Design review of the part built by this model. Coordinates are the model's own, in mm. Give positions to 0.01 mm unless a question says otherwise; leave off trailing zeros. Order: outer loops, then holes, each group sorted by start corner. A loop starts at its lowest first (then second) coordinate and runs counter-clockwise, first axis right, second up. Notation, with made-up numbers: (-4, -25.75) -> (5, -25.75) arc R26 cw to (5, -11.75) -> close; hole circle Ø8 at (72.25, 59.5). An arc over 180 degrees is marked (long way). Return JSON: item names as keys, results as strings.
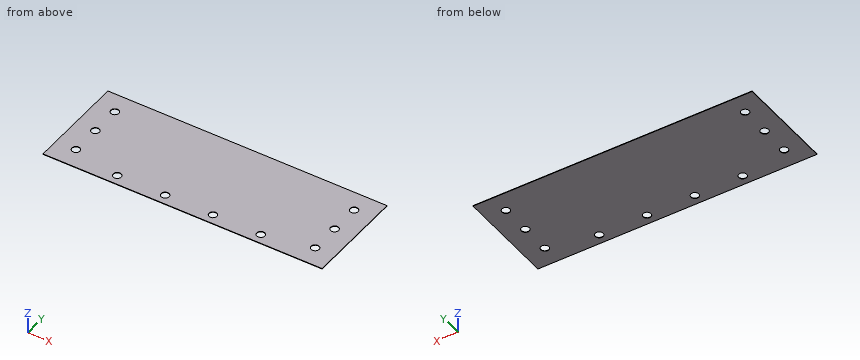
Autodesk Inventor part; units mm, degrees
ref_plane "YZ Plane" through (0, 0, 0) normal (1, 0, 0) x (0, 1, 0)
ref_plane "XZ Plane" through (0, 0, 0) normal (0, 1, 0) x (-1, 0, 0)
ref_plane "XY Plane" through (0, 0, 0) normal (0, 0, 1) x (1, 0, 0)
sketch "Sketch1" plane through (0, 0, 0) normal (0, 0, 1) x (1, 0, 0)
  line L0 (-140, 30) -> (-140, 130)
  line L1 (-140, 130) -> (0, 130)
  line L2 (0, 130) -> (0, 0) construction
  line L3 (140, 30) -> (140, 130)
  line L4 (140, 130) -> (0, 130)
  line L5 (-140, 30) -> (-100, 30)
  line L6 (100, 30) -> (140, 30)
  line L7 (-100, 130) -> (-100, 30)
  line L8 (100, 130) -> (100, 30)
  line L9 (-100, 30) -> (100, 30)
  point P0 (-100, 30)
  point P1 (100, 30)
  dimension "d0" = 140
  dimension "d57" = 40
  dimension "d58" = 40
  dimension "d88" = 100
extrude "Plate3" add sketch "Sketch1" along normal blind 0.5
sketch "Sketch7" plane through (0, 0, 0.5) normal (0, 0, 1) x (1, 0, 0)
  line L0 (-140, 130) -> (140, 130)
  line L1 (-140, 30) -> (-140, 130)
  line L2 (140, 130) -> (140, 30)
  point P0 (0, 0)
  point P1 (-120, 110)
  point P2 (-120, 80)
  point P3 (-120, 50)
  point P4 (120, 110)
  point P5 (120, 80)
  point P6 (120, 50)
  dimension "d98" = 20
  dimension "d99" = 50
  dimension "d100" = 80
  dimension "d101" = 20
  dimension "d102" = 20
  dimension "d103" = 50
  dimension "d104" = 80
  dimension "d105" = 20
hole "Hole6" at (-120, 110, 0.5) at (-120, 80, 0.5) at (-120, 50, 0.5) at (120, 110, 0.5) at (120, 80, 0.5) at (120, 50, 0.5) direction (0, 0, -1) diameter 8 end through all
sketch "Sketch8" plane through (0, 0, 0.5) normal (0, 0, 1) x (1, 0, 0)
  line L0 (0, -26) -> (0, 156)
  line L1 (140, 30) -> (-140, 30)
  point P0 (0, 0)
  point P1 (-72, 40)
  point P2 (-24, 40)
  point P3 (24, 40)
  point P4 (72, 40)
  dimension "d117" = 24
  dimension "d118" = 48
  dimension "d119" = 48
  dimension "d120" = 48
  dimension "d121" = 10
hole "Hole7" at (-72, 40, 0.5) at (-24, 40, 0.5) at (24, 40, 0.5) at (72, 40, 0.5) direction (0, 0, -1) diameter 8 end through all
equation "\"d96\" = Thickness"
equation "\"d111\" = Thickness"
equation "\"d90\" = Thickness"
equation "\"BendRadius\" = Thickness"
equation "\"BendReliefWidth\" = Thickness"
equation "\"BendReliefDepth\" = 0.5 * Thickness"
equation "\"CornerReliefSize\" = 4 * Thickness"
equation "\"MinimumRemnant\" = 2 * Thickness"
equation "\"TransitionRadius\" = BendRadius"
equation "\"JacobiRadiusSize\" = BendRadius"
equation "\"GapSize\" = Thickness"
properties part number "New side"
Item 1: Add section B-B (x = -24). Give the boundary of the cut face in (y, z).
Result set:
{"outline": "(30, 0) -> (36, 0) -> (36, 0.5) -> (30, 0.5) -> close; (44, 0) -> (130, 0) -> (130, 0.5) -> (44, 0.5) -> close"}
Item 2: Add section D-D (x = -120). Give the boundary of the cut face in (y, z).
Result set:
{"outline": "(30, 0) -> (46, 0) -> (46, 0.5) -> (30, 0.5) -> close; (54, 0) -> (76, 0) -> (76, 0.5) -> (54, 0.5) -> close; (84, 0) -> (106, 0) -> (106, 0.5) -> (84, 0.5) -> close; (114, 0) -> (130, 0) -> (130, 0.5) -> (114, 0.5) -> close"}
Item 3: Add section C-C (z = 0.15). Give the number of separate pieces and of enclosed holes in the cut face, plus the area to 3 significant figures.
Result set:
{"separate pieces": "1", "enclosed holes": "10", "area": "27,500 mm^2"}
Item 4: Wall thickness on L1, parallel to Y at x = -120, z = 0.35; L2, parallel to X at y = 40, z = 0.1; L3, parallel to X at y = 110, z = 0.3: over which ranges is each line inside the solid? List them lowest first. Write a range as [from, to].
Result set:
{"L1": "y = [30, 46], [54, 76], [84, 106], [114, 130]", "L2": "x = [-140, -76], [-68, -28], [-20, 20], [28, 68], [76, 140]", "L3": "x = [-140, -124], [-116, 116], [124, 140]"}
Item 5: For pin 1 (13 mm diameter, centred on x = 24, y = 40, fed in from -Z); pin 2 (7 mm diameter, centred on x = -72, y = 40, fed in from -Z), all flat-tipped, find the tip position at first contact; note any pin that passes through.
Result set:
{"pin 1": "stops at z = 0", "pin 2": "passes through"}
Item 6: Add section A-A (y = 80). Give the boundary of the cut face in (x, z), plus the area to 3 significant figures.
Result set:
{"outline": "(-140, 0) -> (-124, 0) -> (-124, 0.5) -> (-140, 0.5) -> close; (-116, 0) -> (116, 0) -> (116, 0.5) -> (-116, 0.5) -> close; (124, 0) -> (140, 0) -> (140, 0.5) -> (124, 0.5) -> close", "area": "132 mm^2"}
